Design review of the part built by this model. Coordinates are the model's own, in mm. Coordinates: 2 decimals unless noted, no trailing zeros.
from build123d import *

# Parameters (mm, degrees)
BOSS_EXTRUDE1_DEPTH = 10.16


with BuildPart() as part:
    # Sketch1 → Boss-Extrude1 (new body)
    with BuildSketch(Plane(origin=(0, 0, 0), x_dir=(0, 0, -1), z_dir=(1, 0, 0))):
        with BuildLine():
            Line((-53.975, -36.5125), (53.975, -36.5125))
            Line((53.975, -36.5125), (53.975, 30.1625))
            ThreePointArc((53.975, 30.1625), (52.115128061, 34.652628061), (47.625, 36.5125))
            Line((47.625, 36.5125), (43.045928132, 36.5125))
            ThreePointArc((43.045928132, 36.5125), (39.235928132, 32.7025), (35.425928132, 36.5125))
            Line((35.425928132, 36.5125), (-35.425928132, 36.5125))
            ThreePointArc((-35.425928132, 36.5125), (-39.235928132, 32.7025), (-43.045928132, 36.5125))
            Line((-43.045928132, 36.5125), (-47.625, 36.5125))
            ThreePointArc((-47.625, 36.5125), (-52.115128061, 34.652628061), (-53.975, 30.1625))
            Line((-53.975, 30.1625), (-53.975, -36.5125))
        make_face()
    extrude(amount=BOSS_EXTRUDE1_DEPTH)


solid = part.part
1. To check wall thickness, follow line 1 (Y direction, x = 5, z = -39); line 2 (Y direction, x = 7, z = 42.5). State the ranges of each line that lie inside material, in increasing order.
2. Insertion check: pin 1 (3 mm diameter, centred on y = -13.5, z = 8.5, fed in from -X). The pin has a flat end and moves straight along its axis. Give the tip position at first contact, or say it passes through.
3. Mouldability with a two-part tool opening along Z and no side actions: class faces 1 (the flat face through (5, 36.512, 45)), 2 (the flat face through (5, -4, -53.975)), 3 (the cylindrical face through (5.009, 32.703, -39.32)) as pulls with the +Z half, pulls with the -Z half, needs draft (parallel to the pull), parting line crosses it, or undercut.
Solution:
1. line 1: y = -36.51 to 32.71
1. line 2: y = -36.51 to 34.55
2. pin 1: stops at x = 0
3. face 1: needs draft
3. face 2: pulls with the -Z half
3. face 3: undercut
